Here's how the part is built. I have some questions about the finished solid (model axes, mm). Face numbers are marked on the shaded views. A direction names the side the tool comes from. Coordinates: 2 decimals unless noted, no trailing zeros. Order: outer loops, then holes, each group sorted by start corner. A loop starts at its lowest first (then second) coordinate and runs counter-clockwise, first axis right, second up. Notation, with made-up numbers: (-20, 48) - (25, 48) arc R22 ccw to (25, 60) - close; hole circle Ø9 at (73.5, 0.25). An arc over 180 degrees is marked (long way). Answer as CSV lines item,"result". Start each with the question number.
Q1. Thinking about a two-plate mould opening in X: for the marked faces 4, 5, 6 and 7, which applies, released by +X, released by -X, zero draft, split by the parting line, or undercut?
Q2. Suppose I cut it at B-B (x = 102.5). Please give me the cut outline in (y, z), then the cut area to 4 significant figures.
Q3. For the marked faces 1, 2 and 3, which set-ups out of +Z, -Z, +X, -X, +Y, -Y let a thin tool reach every point of the face, with its end or its side?
Q4. I need wall thicknesses on line 1 (Y direction, x = 120, z = 33); line 2 (X direction, y = 80, z = 34); line 3 (Z direction, x = 70, y = 13). Which ranges of each line are inside material? Lowest first, please.
Q5. For pin 1 Ø4.5 at (y, z) = (83, 4.5) entering from -X; pin 2 Ø24 at (x, y) = (122.5, 25.5) entering from -Z; pin 3 Ø7.5 at (y, z) = (86, 8) entering from +X; pin 4 Ø1.5 at (y, z) = (80, 2.5) entering from -X, each with a flat end and sliding along its axis, tell me the tip position at first contact or that it passes through.
Q6. Suppose I cut it at C-C (y = 20). Please give me the cut outline in (x, z).
Q7. Suppose I cut it at D-D (z = 24.5). Please give me the cut outline in (x, y), then the cut area to 3 significant figures.
Q8. Suppose I cut it at A-A (z = 49). Please give me the cut outline in (x, y).
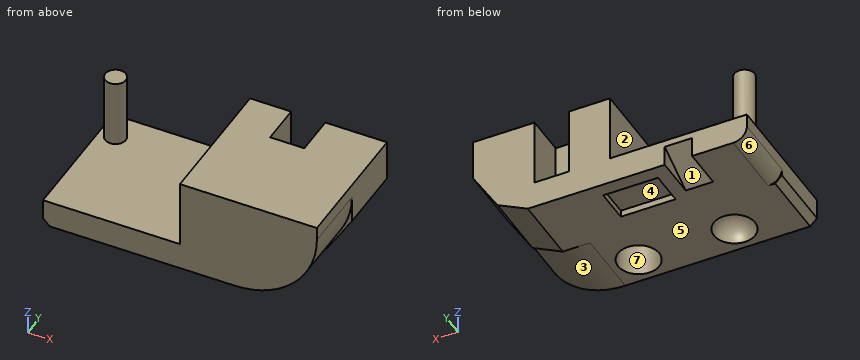
from build123d import *

# Parameters (mm, degrees)
SKICA1_W                 = 200
SKICA1_H                 = 100
P_IDAT_VYSUNUT_M1_DEPTH  = 20
P_IDAT_VYSUNUT_M2_DEPTH  = 50
SKICA7_R                 = 7.5
P_IDAT_VYSUNUT_M3_DEPTH  = 50
ODEBRAT_VYSUNUT_M3_DEPTH = 10
ZAOBLIT1_START           = 50
ZAOBLIT1_DEPTH           = 51
SKICA9_W                 = 40
SKICA9_H                 = 25
ODEBRAT_VYSUNUT_M4_DEPTH = 5
CHAMFER2_SIZE            = 5
FILLET2_DEPTH            = 50
CHAMFER3_SIZE            = 40
CHAMFER3_SIZE2           = 20
CHAMFER4_SIZE            = 20
SKETCH3_R                = 15
CUT_EXTRUDE2_DEPTH       = 60


with BuildPart() as part:
    # Skica1 → Přidat vysunutím1 (new body)
    with BuildSketch(Plane.XY):
        with Locations((100, 50)):
            Rectangle(SKICA1_W, SKICA1_H)
    extrude(amount=P_IDAT_VYSUNUT_M1_DEPTH)

    # Skica2 → Přidat vysunutím2 (add)
    with BuildSketch(Plane.XY.offset(20)):
        Polygon((100, 0), (200, 0), (200, 100), (155, 100), (155, 70), (130, 70), (130, 100), (100, 100), align=None)
    extrude(amount=P_IDAT_VYSUNUT_M2_DEPTH)

    # Skica7 → Přidat vysunutím3 (add)
    with BuildSketch(Plane.XY.offset(20)):
        with Locations(Location((12, 80, 0), (0, 0, 180))):
            Circle(SKICA7_R)
    extrude(amount=P_IDAT_VYSUNUT_M3_DEPTH)

    # Skica8 → Odebrat vysunutím3 (cut, symmetric)
    with BuildSketch(Plane.ZY.offset(-50)):
        Polygon((0, 100), (0, 70), (15, 100), align=None)
    extrude(amount=ODEBRAT_VYSUNUT_M3_DEPTH, both=True, mode=Mode.SUBTRACT)

    # Zaoblit1: read off the stored shape, not the designer's step
    # Zaoblit1 outline → Zaoblit1 (cut)
    with BuildSketch(Plane(origin=(0, 0, 0), x_dir=(1, 0, 0), z_dir=(0, 1, 0)).offset(ZAOBLIT1_START)):
        with BuildLine():
            ThreePointArc((0, -10), (2.928932188, -2.928932188), (10, 0))
            Line((10, 0), (0, 0))
            Line((0, 0), (0, -10))
        make_face()
    extrude(amount=ZAOBLIT1_DEPTH, mode=Mode.SUBTRACT)

    # Skica9 → Odebrat vysunutím4 (cut)
    with BuildSketch(Plane(origin=(0, 0, 0), x_dir=(-1, 0, 0), z_dir=(0, 0, -1))):
        with Locations((-90, 77.5)):
            Rectangle(SKICA9_W, SKICA9_H)
    extrude(amount=-ODEBRAT_VYSUNUT_M4_DEPTH, mode=Mode.SUBTRACT)

    # Chamfer2
    chamfer2_edges = [part.edges().sort_by_distance(p)[0] for p in [
        (0, 25, 0),
    ]]
    chamfer(chamfer2_edges, length=CHAMFER2_SIZE)

    # Fillet2: read off the stored shape, not the designer's step
    # Fillet2 outline → Fillet2 (cut)
    with BuildSketch(Plane(origin=(0, 0, 0), x_dir=(1, 0, 0), z_dir=(0, 1, 0))):
        with BuildLine():
            Line((200, 0), (140, 0))
            ThreePointArc((140, 0), (182.426406871, -17.573593129), (200, -60))
            Line((200, -60), (200, 0))
        make_face()
    extrude(amount=FILLET2_DEPTH, mode=Mode.SUBTRACT)

    # Chamfer3
    chamfer3_edges = [part.edges().sort_by_distance(p)[0] for p in [
        (200, 75, 0),
    ]]
    chamfer3_side = [part.faces().sort_by_distance(p)[0] for p in [
        (93.302047782, 51.38225256, 0),
    ]]
    chamfer(chamfer3_edges, length=CHAMFER3_SIZE, length2=CHAMFER3_SIZE2, reference=chamfer3_side[0])

    # Chamfer4
    chamfer4_edges = [part.edges().sort_by_distance(p)[0] for p in [
        (200, 75, 20),
    ]]
    chamfer(chamfer4_edges, length=CHAMFER4_SIZE)

    # Sketch2 → Cut-Revolve4 (revolve, cut)
    with BuildSketch(Plane(origin=(0, 0, 0), x_dir=(-1, 0, 0), z_dir=(0, 0, -1))):
        with BuildLine():
            Line((-50, 35), (-50, 5))
            ThreePointArc((-50, 5), (-35, 20), (-50, 35))
        make_face()
    revolve(axis=Axis((50, 35, 0), (0, -1, 0)), mode=Mode.SUBTRACT)

    # Sketch3 → Cut-Extrude2 (cut)
    with BuildSketch(Plane(origin=(0, 0, 0), x_dir=(-1, 0, 0), z_dir=(0, 0, -1))):
        with Locations((-120, 20)):
            Circle(SKETCH3_R)
    extrude(amount=-CUT_EXTRUDE2_DEPTH, mode=Mode.SUBTRACT)


solid = part.part
Here are the results:
1,face 4,"undercut"
1,face 5,"zero draft"
1,face 6,"released by -X"
1,face 7,"undercut"
2,outline,"(0, 0) - (65, 0) - (65, 5) - (90, 5) - (90, 0) - (100, 0) - (100, 70) - (0, 70) - close"
2,area,"6,875 mm²"
3,face 1,"-Z, +Y"
3,face 2,"+Z, +Y, -Y"
3,face 3,"-Z, +X, -Y"
4,line 1,"y = 0 to 5, 35 to 100"
4,line 2,"x = 4.5 to 19.5, 100 to 130, 155 to 196.29"
4,line 3,"z = 0 to 20"
5,pin 1,"stops at x = 0.54"
5,pin 2,"stops at z = 0"
5,pin 3,"stops at x = 182.54"
5,pin 4,"stops at x = 2.62"
6,outline,"(0, 5) - (5, 0) - (35, 0) arc R15 cw to (65, 0) - (105, 0) - (105, 60) - (135, 60) - (135, 0) - (140, 0) arc R60 ccw to (200, 60) - (200, 70) - (100, 70) - (100, 20) - (0, 20) - close"
7,outline,"circle Ø15 at (12, 80); (100, 0) - (188.37, 0) - (188.37, 50) - (190.42, 50) - (190.42, 100) - (155, 100) - (155, 70) - (130, 70) - (130, 100) - (100, 100) - close; hole circle Ø30 at (120, 20)"
7,area,"7,660 mm²"
8,outline,"circle Ø15 at (12, 80); (100, 0) - (198.98, 0) - (198.98, 50) - (200, 50) - (200, 100) - (155, 100) - (155, 70) - (130, 70) - (130, 100) - (100, 100) - close; hole circle Ø30 at (120, 20)"
